from build123d import *

# Parameters (mm, degrees)
SKETCH_1_R          = 15
SKETCH_1_R_2        = 7
EXTRUDE_1_DEPTH     = 20
SKETCH_2_R          = 28.5
SKETCH_2_R_2        = 7
EXTRUDE_2_DEPTH     = 5
SKETCH_3_R          = 2.5
CUT_EXTRUDE_1_DEPTH = 5
SKETCH_4_R          = 3
CUT_EXTRUDE_2_DEPTH = 20


with BuildPart() as part:
    # 草图1 → 凸台-拉伸1 (new body)
    with BuildSketch(Plane.XY):
        Circle(SKETCH_1_R)
        Circle(SKETCH_1_R_2, mode=Mode.SUBTRACT)
    extrude(amount=EXTRUDE_1_DEPTH)

    # 草图2 → 凸台-拉伸2 (add)
    with BuildSketch(Plane.XY.offset(20)):
        Circle(SKETCH_2_R)
        Circle(SKETCH_2_R_2, mode=Mode.SUBTRACT)
    extrude(amount=EXTRUDE_2_DEPTH)

    # 草图3 → 切除-拉伸1 (cut)
    with BuildSketch(Plane.XY.offset(25)):
        with Locations((0, -24)):
            Circle(SKETCH_3_R)
        with Locations((-16.970562748, -16.970562748)):
            Circle(SKETCH_3_R)
        with Locations((-24, 0)):
            Circle(SKETCH_3_R)
        with Locations((-16.970562748, 16.970562748)):
            Circle(SKETCH_3_R)
        with Locations((0, 24)):
            Circle(SKETCH_3_R)
        with Locations((16.970562748, 16.970562748)):
            Circle(SKETCH_3_R)
        with Locations((24, 0)):
            Circle(SKETCH_3_R)
        with Locations((16.970562748, -16.970562748)):
            Circle(SKETCH_3_R)
    extrude(amount=-CUT_EXTRUDE_1_DEPTH, mode=Mode.SUBTRACT)

    # 草图4 → 切除-拉伸2 (cut)
    with BuildSketch(Plane(origin=(0, 0, 0), x_dir=(1, 0, 0), z_dir=(0, 1, 0))):
        with Locations(Location((0, -10, 0), (0, 0, 270))):
            Circle(SKETCH_4_R)
    extrude(amount=-CUT_EXTRUDE_2_DEPTH, mode=Mode.SUBTRACT)


solid = part.part
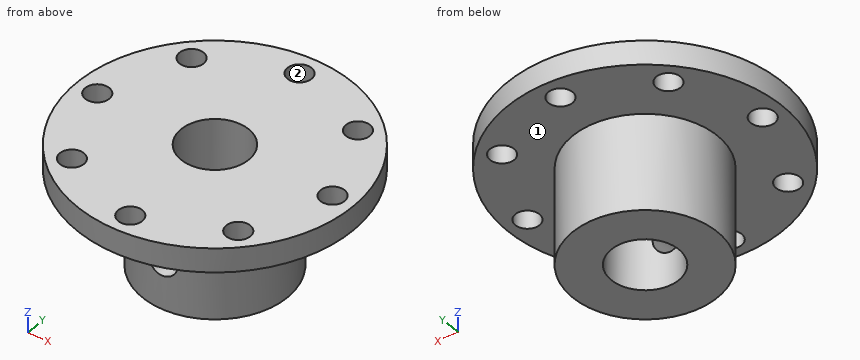
Read the model definition and answer for the solid it produces. Units are mm, in the model's axes. Face numbers are marked on the shaded views. A direction names the side the tool comes from. Round coordinates to 2 decimals unless told otherwise and drop trailing zeros. Write each loop counter-clockwise with the first axis right and the second up, starting at its lowest first coordinate (ties: lowest second). Pieces come first, ordered by that corner, then holes. Notation, with made-up numbers: (12, -23) - (46, -23) arc R23 ccw to (46, -1) - close; hole circle Ø4 at (43.25, 48.25). An arc over 180 degrees is marked (long way). One line per question, with ' | ' between items. Start each with the question number.
1. Section C-C (y = -10) is taken. Determine the outline of the cut face in (x, z).
2. Section A-A (x = 0) is taken. Determine the outline of the cut face in (y, z).
3. Find the intervals of material crossed by probe 1 along Y at (x, z) = (0, 22.15); probe 2 along Z at (x, y) = (-17, 20.5); probe 3 along Y at (x, z) = (-24, 22.7), in increasing order. Write a range as [from, to].
4. For the marked faces 1 and 2, determine the directions among +Z, -Z, +X, -X, +Y, -Y from which every point of the face is accessible in a straight line to the end or side of a thin tool.
5. Section D-D (z = 13.75) is taken. Determine the outline of the cut face in (x, y), and give its area (3 significant figures).
6. Section B-B (y = -4) is taken. Determine the outline of the cut face in (x, z).
7. Each of these flat-tipped pins is pushed along its axis until it touches: pin 1 (6.5 mm diameter, centred on x = 16.97, y = -16.97, fed in from -Z); pin 2 (3 mm diameter, centred on y = 7.5, z = 8, fed in from +X); pin 3 (4 mm diameter, centred on x = -16.97, y = 16.97, fed in from +Z); pin 4 (8 mm diameter, centred on x = 0, z = 10, fed in from -Y). Where does it stop, or does it pass through?
Filled in:
1) outline: (-26.69, 20) - (-11.18, 20) - (-11.18, 0) - (11.18, 0) - (11.18, 20) - (26.69, 20) - (26.69, 25) - (-26.69, 25) - close; hole circle Ø6 at (0, 10)
2) outline: (-28.5, 20) - (-26.5, 20) - (-26.5, 25) - (-28.5, 25) - close; (-21.5, 20) - (-15, 20) - (-15, 13) - (-7, 13) - (-7, 25) - (-21.5, 25) - close; (-15, 0) - (-7, 0) - (-7, 7) - (-15, 7) - close; (7, 0) - (15, 0) - (15, 20) - (21.5, 20) - (21.5, 25) - (7, 25) - close; (26.5, 20) - (28.5, 20) - (28.5, 25) - (26.5, 25) - close
3) probe 1: [-28.5, -26.5], [-21.5, -7], [7, 21.5], [26.5, 28.5] | probe 2: [20, 25] | probe 3: [-15.37, -2.5], [2.5, 15.37]
4) face 1: -Z | face 2: +Z, -Z
5) outline: circle Ø30 at (0, 0); hole circle Ø14 at (0, 0) | area: 553 mm²
6) outline: (-28.22, 20) - (-14.46, 20) - (-14.46, 0) - (-5.74, 0) - (-5.74, 25) - (-28.22, 25) - close; (5.74, 0) - (14.46, 0) - (14.46, 20) - (28.22, 20) - (28.22, 25) - (5.74, 25) - close
7) pin 1: z = 20 | pin 2: x = 13.75 | pin 3: through | pin 4: y = -15
